The listing builds one solid part. Answer for the finished solid, in the listing's coordinates (mm). A direction names the side the tool comes from. Coordinates: 2 decimals unless noted, no trailing zeros. Loops run counter-clockwise (first coordinate to the right, second up) from the corner with the lowest first, then second, coordinate; pieces in that order, holes last. Notation, with made-up numbers: (-28.5, 8.25) - (7.5, 8.25) arc R6 cw to (7.5, 15.25) - close; hole circle Ø10 at (5, 70). An arc over 180 degrees is marked (long way). Return JSON: item names as keys, results as strings. Group by question number.
1. Section B-B (y = 0) is taken. State how many separate pieces and enclosed holes the cut face has, and give its area (3 significant figures).
2. Section A-A (x = 0) is taken. Write down the section's boundary in (y, z), and give its area (3 significant figures).
3. Which of the six approach directions +Z, -Z, +X, -X, +Y, -Y give full straight-line access (tool end or side, diameter ignored) to faces 4 (the face through (-3.64, 0.08, -4.14)), 5 (the face through (-2, -8, -0.75)), 6 (the face through (0, -5, 8))?
4. The mould has two halves that part along Z. Classify faces 1 (the face through (-3.86, 12.13, -0.52)), 2 (the face through (0, 6, -0.75)), 3 (the face through (-1.03, -6.65, 2.9)): pulls with the +Z half, pulls with the -Z half, needs draft (parallel to the pull), parting line crosses it, or undercut.
5. Find the intervals of material crossed by line 1 along Z through (x, y) = (-1, 0); line 2 along X through (y, z) = (-8, 8.5); line 3 along Z through (x, y) = (1, 1), in increasing order.
6. Section D-D (x = -2.5) is taken. Write down the section's boundary in (y, z), and give its area (3 significant figures).
7. Each of these flat-tipped pins is pushed along its axis until it touches: P1, Ø1.2, axis at x = 1.5, z = 0, coming from the -Y side; P2, Ø1.2, axis at x = 0, y = 5.5, coming from the +Z side; P3, Ø3, axis at x = 1, y = -7, coming from the +Z side. Where does it stop, or does it pass through?
Autodesk Inventor part; units mm, degrees
ref_plane "body_screw_XY" through (0, -8, 5) normal (0, 0, 1) x (1, 0, 0)
ref_plane "body_screw_YZ" through (0, -8, 5) normal (1, 0, 0) x (0, 1, 0)
ref_plane "body_screw_ZX" through (0, -8, 5) normal (0, 1, 0) x (0, 0, 1)
sketch "Sketch_1" plane through (0, 0, 0) normal (0, 0, 1) x (1, 0, 0)
  line L0 (4, 0) -> (-4, 0)
  line L1 (-4, 12) -> (-4, 4.5)
  line L2 (-4, 4.5) -> (-3.5, 4)
  line L3 (-3.5, 4) -> (3.5, 4)
  line L4 (3.5, 4) -> (4, 4.5)
  line L5 (4, 4.5) -> (4, 12)
  line L6 (4, 12) -> (3.5, 12.5)
  line L7 (3.5, 12.5) -> (-3.5, 12.5)
  line L8 (-3.5, 12.5) -> (-4, 12)
revolve "Revolution1" add sketch "Sketch_1" angle 360 about axis through (4, 0, 0) along (1, 0, 0)
sketch "Sketch_2" plane through (0, 0, 0) normal (1, 0, 0) x (0, 1, 0)
  line L0 (-12.5, 0.75) -> (-12.5, -0.75)
  line L1 (-12.5, -0.75) -> (8, -0.75)
  line L2 (8, -0.75) -> (8, 0.75)
  line L3 (8, 0.75) -> (-12.5, 0.75)
extrude "Extrusion1" cut sketch "Sketch_2" along normal mid plane 8
sketch "Sketch_3" plane through (0, 0, 0) normal (1, 0, 0) x (0, 1, 0)
  line L0 (-8, 12.5) -> (-8, 0)
  line L1 (-8, 0) -> (-9.7, 0)
  line L2 (-9.7, 0) -> (-9.7, 5)
  line L3 (-9.7, 5) -> (-11, 5)
  line L4 (-11, 5) -> (-11, 12.5)
  line L5 (-11, 12.5) -> (-8, 12.5)
  line L6 (-8, 12.5) -> (-8, 0)
revolve "Revolution2" cut sketch "Sketch_3" angle 360 about axis through (0, -8, 12.5) along (0, 0, 1)
sketch "Sketch_4" plane through (0, 0, 0) normal (1, 0, 0) x (0, 1, 0)
  line L0 (-8, -12.75) -> (-8, -0.75)
  line L1 (-8, -0.75) -> (-6.5, -0.75)
  line L2 (-6.5, -0.75) -> (-6.7705, -1.0205)
  line L3 (-6.7705, -1.0205) -> (-6.7705, -12.75)
  line L4 (-6.7705, -12.75) -> (-8, -12.75)
  line L5 (-8, -12.75) -> (-8, -0.75)
revolve "Revolution3" cut sketch "Sketch_4" angle 360 about axis through (0, -8, -12.75) along (0, 0, -1)
thread "Thread1"
sketch "Sketch_7" plane through (0, 0, -7) normal (0, 0, 1) x (1, 0, 0)
  line L0 (4, 0) -> (-4, 0)
  line L1 (-4, 0) -> (-4, 1.5)
  line L2 (-4, 1.5) -> (-3.7295, 1.2295)
  line L3 (-3.7295, 1.2295) -> (3.7295, 1.2295)
  line L4 (3.7295, 1.2295) -> (4, 1.5)
  line L5 (4, 1.5) -> (4, 0)
  line L6 (4, 0) -> (-4, 0)
revolve "Revolution4" cut sketch "Sketch_7" angle 360 about axis through (4, 0, -7) along (1, 0, 0)
thread "Thread2"
sketch "Sketch_8" plane through (0, 0, 7) normal (0, 0, 1) x (1, 0, 0)
  line L0 (4, 0) -> (-4, 0)
  line L1 (-4, 0) -> (-4, 1.5)
  line L2 (-4, 1.5) -> (-3.7295, 1.2295)
  line L3 (-3.7295, 1.2295) -> (3.7295, 1.2295)
  line L4 (3.7295, 1.2295) -> (4, 1.5)
  line L5 (4, 1.5) -> (4, 0)
  line L6 (4, 0) -> (-4, 0)
revolve "Revolution5" cut sketch "Sketch_8" angle 360 about axis through (4, 0, 7) along (1, 0, 0)
thread "Thread3"
ref_plane "body_screw_XY" through (0, -8, 5) normal (0, 0, 1) x (1, 0, 0)
ref_plane "body_screw_YZ" through (0, -8, 5) normal (1, 0, 0) x (0, 1, 0)
ref_plane "body_screw_ZX" through (0, -8, 5) normal (0, 1, 0) x (0, 0, 1)
properties part number "SCSWA8-8b"
The answers:
{
 "1": {"separate pieces": "4", "enclosed holes": "0", "area": "95.4 mm2"},
 "2": {"outline": "(-12.48, -0.75) arc R12.5 ccw to (-9.23, -8.43) - (-9.23, -1.02) - (-9.5, -0.75) - close; (-12.48, 0.75) - (-9.7, 0.75) - (-9.7, 5) - (-11, 5) - (-11, 5.94) arc R12.5 ccw to start; (-6.77, -10.51) arc R12.5 ccw (long way) to (-5, 11.46) - (-5, 5) - (-6.3, 5) - (-6.3, 0.75) - (-3.93, 0.75) arc R4 cw to (3.93, 0.75) - (8, 0.75) - (8, -0.75) - (3.93, -0.75) arc R4 cw to (-3.93, -0.75) - (-6.5, -0.75) - (-6.77, -1.02) - close; hole circle Ø2.46 at (0, -7); hole circle Ø2.46 at (0, 7)", "area": "350 mm2"},
 "3": {"face 4": "-X", "face 5": "+X, -X, -Y", "face 6": "+Z"},
 "4": {"face 1": "parting line crosses it", "face 2": "undercut", "face 3": "needs draft"},
 "5": {"line 1": "z = -12.5 to -8.23, -5.77 to -4, 4 to 5.77, 8.23 to 12.5", "line 2": "x = -4 to -3, 3 to 4", "line 3": "z = -12.46 to -7.72, -6.28 to -3.87, 3.87 to 6.28, 7.72 to 12.46"},
 "6": {"outline": "(-12.48, -0.75) arc R12.5 ccw (long way) to (-6.34, 10.77) - (-6.34, 5) - (-9.66, 5) - (-9.66, 7.94) arc R12.5 ccw to (-12.48, 0.75) - (-3.93, 0.75) arc R4 cw to (3.93, 0.75) - (8, 0.75) - (8, -0.75) - (3.93, -0.75) arc R4 cw to (-3.93, -0.75) - close; hole circle Ø2.46 at (0, -7); hole circle Ø2.46 at (0, 7)", "area": "397 mm2"},
 "7": {"P1": "stops at y = 8", "P2": "stops at z = 11.5", "P3": "stops at z = 5"}
}
